Work out the finished part from the listing and answer in its coordinate system (mm). Face numbers are marked on the shaded views. A direction names the side the tool comes from. Round coordinates to 2 decimals unless told otherwise and drop trailing zeros. Write each loop counter-clockwise with the first axis right and the second up, starting at its lowest first coordinate (ties: lowest second). Pieces come first, ordered by that corner, then holes. Notation, with made-up numbers: M 78.25,43.25 L 104.25,43.25 A10 cw 104.25,53.25 Z; hole C -12,-37.5 d6. An arc over 180 degrees is marked long. One line per item, written item: value. Start each with the question number.
Q1. Find section C-C (y = -91). Write down the section's boundary in (x, z) (3 decimals), and give its area (3 significant figures).
Q2. A tool of negligible diameter and unlimited length cuts with its end or side. For the marked faces 1, 2 and 3, from which of +Z, -Z, +X, -X, +Y, -Y can it reach the whole face along a straight path? Write none if from no direction.
Q3. Find section A-A (z = 4.5). Count the separate pieces of the cut face and the enclosed holes in it, and give its area (3 significant figures).
Q4. Given pin 1 Ø4 at (x, y) = (-2.5, -28) entering from -Z; pin 2 Ø2 at (x, y) = (-2, -95.5) entering from -Z; pin 3 Ø3 at (x, z) = (-5, -42.5) entering from +Y, each flat-ended and moving along its own axis, determine where each tip first touches the part or whether it passes through.
Q5. Find section D-D (z = -40.5). Write down the section's boundary in (x, y) (3 decimals).
Q6. Consider probe 1 along Z at (x, y) = (0.5, -14.5) (3 decimals); probe 2 along X at (y, z) = (-101, -44.5); probe 3 along Z at (x, y) = (-3.25, -77). Determine where each line is inside the solid, lowest interval first.
from build123d import *

# Parameters (mm, degrees)
SKETCH5_W           = 12.880016042
SKETCH5_H           = 15.834691301
CUT_EXTRUDE2_DEPTH  = 7.62
CUT_EXTRUDE6_REACH  = 62
SKETCH11_W          = 3.175
SKETCH11_H          = 3.175
BOSS_EXTRUDE1_DEPTH = 6.35
CUT_EXTRUDE4_DEPTH  = 3.175
SKETCH10_W          = 4
SKETCH10_H          = 0.5
CUT_EXTRUDE5_DEPTH  = 37.349999944
CUT_EXTRUDE7_DEPTH  = 40.64
BOSS_EXTRUDE3_DEPTH = 12.7
SKETCH19_W          = 21.319602533
SKETCH19_H          = 36.10119369
CUT_EXTRUDE10_DEPTH = 13.7
SKETCH15_W          = 6.35
SKETCH15_H          = 3.175
BOSS_EXTRUDE2_DEPTH = 1.5875
SKETCH17_W          = 3.175
SKETCH17_H          = 37.332237063
CUT_EXTRUDE9_DEPTH  = 20


with BuildPart() as part:
    # Sketch2 → Revolve1 (revolve)
    with BuildSketch(Plane(origin=(0, 0, 0), x_dir=(0, 0, -1), z_dir=(1, 0, 0))):
        Polygon((0, -50.8), (-29.999999944, 0), (0, 0), align=None)
    revolve(axis=Axis((0, 0, 0), (0, -1, 0)))

    # Sketch4 → Cut-Revolve1 (revolve, cut)
    with BuildSketch(Plane(origin=(0, 0, 0), x_dir=(0, 0, -1), z_dir=(1, 0, 0))):
        Polygon((0, -45.72), (-24.919999944, 0), (0, 0), align=None)
    revolve(axis=Axis((0, 16.11457811, 0), (0, -1, 0)), mode=Mode.SUBTRACT)

    # Sketch5 → Cut-Extrude2 (cut, symmetric)
    with BuildSketch(Plane(origin=(0, 0, 0), x_dir=(0, 0, -1), z_dir=(1, 0, 0))):
        with Locations((0, -47.812265381)):
            Rectangle(SKETCH5_W, SKETCH5_H)
    extrude(amount=CUT_EXTRUDE2_DEPTH, both=True, mode=Mode.SUBTRACT)

    # Sketch11 → Cut-Extrude6 (cut, up to next)
    with BuildSketch(Plane.XY.offset(29.999999944), mode=Mode.PRIVATE) as cut_extrude6_sk1:
        with Locations((4.7625, -1.5875)):
            Rectangle(SKETCH11_W, SKETCH11_H)
    cut_extrude6_tool1 = extrude(cut_extrude6_sk1.sketch, amount=-CUT_EXTRUDE6_REACH, mode=Mode.PRIVATE) & part.part
    add(cut_extrude6_tool1.solids().sort_by_distance((4.7625, -1.5875, 30))[0], mode=Mode.SUBTRACT)
    # Sketch11 → Cut-Extrude6 (cut, up to next)
    with BuildSketch(Plane.XY.offset(29.999999944), mode=Mode.PRIVATE) as cut_extrude6_sk2:
        with Locations((-4.7625, -1.5875)):
            Rectangle(SKETCH11_W, SKETCH11_H)
    cut_extrude6_tool2 = extrude(cut_extrude6_sk2.sketch, amount=-CUT_EXTRUDE6_REACH, mode=Mode.PRIVATE) & part.part
    add(cut_extrude6_tool2.solids().sort_by_distance((-4.7625, -1.5875, 30))[0], mode=Mode.SUBTRACT)

    # Sketch6 → Boss-Extrude1 (add, symmetric)
    with BuildSketch(Plane(origin=(0, 0, 0), x_dir=(0, 0, -1), z_dir=(1, 0, 0))):
        with BuildLine():
            Line((0, -39.89491973), (-7.374618631, -39.89491973))
            Line((-7.374618631, -39.89491973), (11.56279342, -71.962270863))
            ThreePointArc((11.56279342, -71.962270863), (29.890602823, -92.707185326), (54.61, -105.165575141))
            ThreePointArc((54.61, -105.165575141), (64.513552335, -107.250553005), (74.61, -107.95))
            Line((74.61, -107.95), (77.785, -107.95))
            Line((77.785, -107.95), (77.785, -100.0125))
            Line((77.785, -100.0125), (74.61, -100.0125))
            Line((74.61, -100.0125), (74.61, -101.6))
            ThreePointArc((74.61, -101.6), (41.460280796, -92.804941633), (17.03053379, -68.733290336))
            Line((17.03053379, -68.733290336), (0, -39.89491973))
        make_face()
        Polygon((-30.934610553, 0), (-7.374618631, -39.89491973), (0, -39.89491973), (-23.559991923, 0), align=None)
    extrude(amount=BOSS_EXTRUDE1_DEPTH, both=True)

    # Sketch7 → Cut-Extrude4 (cut)
    with BuildSketch(Plane(origin=(0, 0, 0), x_dir=(0, 0, -1), z_dir=(1, 0, 0))):
        with BuildLine():
            Line((-3.175, -39.89491973), (14.676503495, -70.123465704))
            ThreePointArc((14.676503495, -70.123465704), (36.599939349, -93.039017482), (66.414189392, -103.849662572))
            ThreePointArc((66.414189392, -103.849662572), (70.51080038, -104.32379518), (74.61, -104.775))
            Line((74.61, -104.775), (74.61, -101.6))
            ThreePointArc((74.61, -101.6), (59.345071166, -99.83437787), (44.886242604, -94.630749287))
            ThreePointArc((44.886242604, -94.630749287), (29.078331812, -83.704237641), (17.03053379, -68.733290336))
            Line((17.03053379, -68.733290336), (-23.559991923, 0))
            Line((-23.559991923, 0), (-26.734991923, 0))
            Line((-26.734991923, 0), (-3.175, -39.89491973))
        make_face()
    cut_extrude4 = extrude(amount=-CUT_EXTRUDE4_DEPTH, mode=Mode.SUBTRACT)

    # Mirror1: Cut-Extrude4 across plane
    add(cut_extrude4.mirror(Plane(origin=(0, 0, 0), x_dir=(0, 0, 1), z_dir=(1, 0, 0))), mode=Mode.SUBTRACT)

    # Sketch9 → Cut-Revolve2 (revolve, cut)
    with BuildSketch(Plane(origin=(0, 0, 0), x_dir=(0, 0, -1), z_dir=(1, 0, 0))):
        Polygon((0, 0), (-24.9199908, 0), (-0.536470716, -39.89491973), (0, -39.89491973), align=None)
    revolve(axis=Axis((0, 16.11457811, 0), (0, -1, 0)), mode=Mode.SUBTRACT)

    # Sketch10 → Cut-Extrude5 (cut, through all)
    with BuildSketch(Plane.ZY.offset(6.35)):
        with BuildLine():
            Line((-70.61, -104.775), (-70.61, -101.480258272))
            ThreePointArc((-70.61, -101.480258272), (-72.609104071, -101.570057864), (-74.61, -101.6))
            Line((-74.61, -101.6), (-74.61, -104.775))
            Line((-74.61, -104.775), (-70.61, -104.775))
        make_face()
        with Locations((-72.61, -105.025)):
            Rectangle(SKETCH10_W, SKETCH10_H)
    extrude(amount=-CUT_EXTRUDE5_DEPTH, mode=Mode.SUBTRACT)

    # Sketch12 → Cut-Extrude7 (cut, symmetric)
    with BuildSketch(Plane.ZY):
        Polygon((30, 0), (-61.025869449, 0), (-61.025869449, -39.89491973), (-6.440008021, -39.89491973), (6.44000802, -39.89491973), (27.945214206, -3.175), align=None)
    extrude(amount=CUT_EXTRUDE7_DEPTH, both=True, mode=Mode.SUBTRACT)

    # Sketch18 → Boss-Extrude3 (add)
    with BuildSketch(Plane.ZY.offset(6.35)):
        with BuildLine():
            Line((6.44000802, -39.89491973), (6.44000802, 0))
            Line((6.44000802, 0), (9.61500802, 0))
            Line((9.61500802, 0), (9.61500802, -34.473639686))
            Line((9.61500802, -34.473639686), (9.61500802, -36.10119369))
            ThreePointArc((9.61500802, -36.10119369), (8.57844205, -39.89491973), (5.756782033, -42.634456374))
            Line((5.756782033, -42.634456374), (6.44000802, -41.477527034))
            Line((6.44000802, -41.477527034), (6.44000802, -39.89491973))
        make_face()
    extrude(amount=-BOSS_EXTRUDE3_DEPTH)

    # Sketch19 → Cut-Extrude10 (cut, through all)
    with BuildSketch(Plane.ZY.offset(6.35)):
        with Locations((20.274809287, -18.050596845)):
            Rectangle(SKETCH19_W, SKETCH19_H)
    extrude(amount=-CUT_EXTRUDE10_DEPTH, mode=Mode.SUBTRACT)

    # Sketch15 → Boss-Extrude2 (add, symmetric)
    with BuildSketch(Plane.ZY.offset(6.35)):
        with Locations((6.44000802, -1.5875)):
            Rectangle(SKETCH15_W, SKETCH15_H)
    boss_extrude2 = extrude(amount=BOSS_EXTRUDE2_DEPTH, both=True)

    # Mirror2: Boss-Extrude2 across plane
    add(boss_extrude2.mirror(Plane(origin=(0, 0, 0), x_dir=(0, 0, 1), z_dir=(1, 0, 0))))

    # Sketch17 → Cut-Extrude9 (cut)
    with BuildSketch(Plane(origin=(0, 0, -77.785), x_dir=(-1, 0, 0), z_dir=(0, 0, -1))):
        with Locations((-4.7625, -89.283881468)):
            Rectangle(SKETCH17_W, SKETCH17_H)
        with Locations((4.7625, -89.283881468)):
            Rectangle(SKETCH17_W, SKETCH17_H)
    extrude(amount=-CUT_EXTRUDE9_DEPTH, mode=Mode.SUBTRACT)


solid = part.part
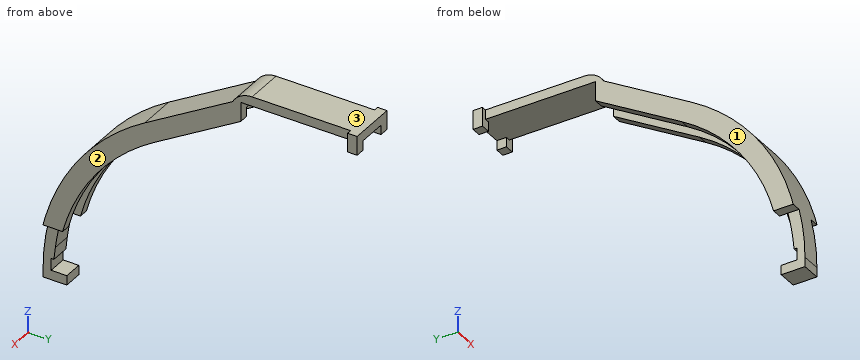
The answers:
1. outline: M -6.35,-38.481 L -3.175,-38.481 L -3.175,-33.642 L 3.175,-33.642 L 3.175,-38.481 L 6.35,-38.481 L 6.35,-27.761 L -6.35,-27.761 Z
1. area: 105 mm2
2. face 1: +Z, -Z, -X, -Y
2. face 2: +Z, -Z, +X, -Y
2. face 3: +Z, +X, -X, +Y, -Y
3. separate pieces: 3
3. enclosed holes: 0
3. area: 82.0 mm2
4. pin 1: z = 6.44
4. pin 2: z = -42.53
4. pin 3: y = -92.54
5. outline: M -6.35,-99.52 L 6.35,-99.52 L 6.35,-92.246 L 3.175,-92.246 L 3.175,-95.403 L -3.175,-95.403 L -3.175,-92.246 L -6.35,-92.246 Z
6. probe 1: 6.44 to 9.615
6. probe 2: -6.35 to 6.35
6. probe 3: -22.79 to -14.82
